Source: CAD feature listing. Evaluate the final solid. Frame: model axes, mm. A direction names the side the tool comes from. Round coordinates to 2 decimals unless told otherwise and drop trailing zeros. Order: outer loops, then holes, each group sorted by start corner. A loop starts at its lowest first (then second) coordinate and runs counter-clockwise, first axis right, second up. Notation, with made-up numbers: (-37, 38.25) - (10, 38.25) arc R22 cw to (10, 61.25) - close; hole circle Ø10 at (30.25, 67.5). An arc over 180 degrees is marked (long way). Return JSON: item names as keys, results as strings. Group by question number.
1) Ray query, line 1 (Y direction, x = 5, z = 67.5) (3 decimals); line 2 (Y direction, x = 6.75, z = 46); line 3 (X direction, y = -21.5, z = 86). Return the intervals inside material, ascending. Write a range as from..to.
2) Section C-C, the plane x = 13. Return loops of the section in (y, z), plus the area to 3 significant figures.
3) Section A-A, the plane z = 85.5. Return loops of the section in (x, y) (3 decimals), plus the area to 3 significant figures.
4) Access query for faces 1 (the cylindrical face through (4.9, -24.5, 59.2)), 2 (the flat face through (11, 7, 25)). Directions: +Z, -Z, +X, -X, +Y, -Y. A direction counts if a zero-diameter tool reaches every point of the face in a straight line with its end or side. Return the directions, or none.
5) Section D-D, the plane y = -12.5. Return loops of the section in (x, z), plus the area to 3 significant figures.
6) Contact query for flat-ended pins moving along their axis: P1, Ø8, axis at x = 14, y = 6, coming from the -Z side; P2, Ø4, axis at y = -2.5, z = 15.5, coming from the -X side; P3, Ø4, axis at x = 16.5, z = 93.5, coming from the -Y side. Output: stop coordinate, or through.
7) Mould query, pull axis Y, two halves, no side actions, for faces 3 (the flat face through (-1.963, -10.429, 59.16)), 4 (the cylindrical face through (2.5, 0.8, 59.2)), 5 (the flat face through (21.541, 6, 72)). Classes: pulls with the +Y half, pulls with the -Y half, needs draft (parallel to the pull), parting line crosses it, or undercut.
8) Section B-B, the plane y = 0. Return loops of the section in (x, z) (3 decimals).
```python
from build123d import *

# Parameters (mm, degrees)
ESQUISSE1_R             = 2.625
BOSS_EXTRU_1_DEPTH      = 120
ENL_V_MAT_EXTRU_1_DEPTH = 25


with BuildPart() as part:
    # Esquisse1 → Boss.-Extru.1 (new body)
    with BuildSketch(Plane.XY):
        with BuildLine():
            ThreePointArc((-0.79755539, 4.428758901), (-3.787637609, 2.429773929), (-4.358021192, -1.12145053))
            Line((-4.358021192, -1.12145053), (0.5, -20))
            ThreePointArc((0.5, -20), (5, -24.5), (9.5, -20))
            Line((9.5, -20), (11.28572177, -17.287605871))
            ThreePointArc((11.28572177, -17.287605871), (10.940890985, -17.183131081), (10.599214607, -17.068761049))
            ThreePointArc((10.599214607, -17.068761049), (2.237966256, -5.391928791), (10.376689651, 6.441078731))
            ThreePointArc((10.376689651, 6.441078731), (16.104400227, 7.151408987), (21.540678755, 5.212823607))
            Line((21.540678755, 5.212823607), (21.540678755, 7.531281515))
            ThreePointArc((21.540678755, 7.531281515), (13.221135766, 9.146884287), (5.419576542, 5.836198326))
            Line((5.419576542, 5.836198326), (-0.79755539, 4.428758901))
        make_face()
        with Locations((5, -20)):
            Circle(ESQUISSE1_R, mode=Mode.SUBTRACT)
        Circle(ESQUISSE1_R, mode=Mode.SUBTRACT)
    extrude(amount=BOSS_EXTRU_1_DEPTH)

    # Esquisse2 → Enlèv. mat.-Extru.1 (cut)
    with BuildSketch(Plane(origin=(0, 0, 0), x_dir=(-1, 0, 0), z_dir=(0, 0, -1))):
        with BuildLine():
            Line((-0.802648586, 4.838533405), (-23.542155856, 15.333417872))
            Line((-23.542155856, 15.333417872), (-23.542155856, 4.140650018))
            Line((-23.542155856, 4.140650018), (-4.513818825, 1.918616657))
            ThreePointArc((-4.513818825, 1.918616657), (-3.032768518, 3.854603141), (-0.802648586, 4.838533405))
        make_face()
    extrude(amount=-ENL_V_MAT_EXTRU_1_DEPTH, mode=Mode.SUBTRACT)


solid = part.part
```
Geometry check:
{
 "1": {"line 1": "-24.5..-22.625, -17.375..-13.112, 2.564..5.741", "line 2": "-24.15..-21.96, -18.04..-14.89, 4.34..6.83", "line 3": "0.76..2.85, 7.15..9.24"},
 "2": {"outline": "(7.11, 25) - (9.12, 25) - (9.12, 120) - (7.11, 120) - close", "area": "192 mm2"},
 "3": {"outline": "(-4.358, -1.121) - (0.5, -20) arc R4.5 ccw to (9.5, -20) - (11.286, -17.288) arc R12.5 cw (long way) to (21.541, 5.213) - (21.541, 7.531) arc R14.5 ccw to (5.42, 5.836) - (-0.798, 4.429) arc R4.5 ccw to start; hole circle Ø5.25 at (0, 0); hole circle Ø5.25 at (5, -20)", "area": "203 mm2"},
 "4": {"face 1": "+Z, -Z, -Y", "face 2": "-Z, +X, +Y"},
 "5": {"outline": "(-1.43, 0) - (4.54, 0) - (4.54, 120) - (-1.43, 120) - close", "area": "716 mm2"},
 "6": {"P1": "z = 25", "P2": "x = -4.47", "P3": "y = 6.65"},
 "7": {"face 3": "pulls with the -Y half", "face 4": "undercut", "face 5": "needs draft"},
 "8": {"outline": "(-4.5, 0) - (-2.625, 0) - (-2.625, 120) - (-4.5, 120) - close; (2.625, 0) - (3.404, 0) - (3.404, 120) - (2.625, 120) - close"}
}
